```python
from build123d import *

# Parameters (mm, degrees)
SKETCH1_R               = 15.875
SKETCH1_R_2             = 9.5
BOSS_EXTRUDE1_DEPTH     = 6
BOSS_EXTRUDE2_START     = 13.050000011
SKETCH2_R               = 15.875
SKETCH2_R_2             = 9.5
SKETCH2_R_3             = 6.35
BOSS_EXTRUDE2_DEPTH     = 13.050000011
SKETCH3_R               = 1.95
CUT_EXTRUDE1_DEPTH      = 10.16
CUT_EXTRUDE3_REACH      = 39.82
CUT_EXTRUDE3_END_RADIUS = 6.35
BOSS_EXTRUDE3_REACH     = 31.444
SKETCH7_R               = 3.15
CUT_EXTRUDE4_DEPTH      = 31.75
CUT_EXTRUDE5_REACH      = 53.87
CUT_EXTRUDE5_END_RADIUS = 3.15
SKETCH8_R               = 1.95
FILLET1_R               = 9.525


with BuildPart() as part:
    # Sketch1 → Boss-Extrude1 (new body)
    with BuildSketch(Plane(origin=(0, 0, 0), x_dir=(0, 0, -1), z_dir=(1, 0, 0))):
        Circle(SKETCH1_R)
        Circle(SKETCH1_R_2, mode=Mode.SUBTRACT)
    extrude(amount=BOSS_EXTRUDE1_DEPTH)

    # Sketch2 → Boss-Extrude2 (add)
    # profile 1 of 2: a face of its own
    with BuildSketch(Plane.ZY.offset(BOSS_EXTRUDE2_START)):
        Circle(SKETCH2_R)
        with Locations(Location((0, 0, 0), (0, 0, 180))):
            Circle(SKETCH2_R_2, mode=Mode.SUBTRACT)
    # profile 2 of 2: a face of its own
    with BuildSketch(Plane.ZY.offset(BOSS_EXTRUDE2_START)):
        with Locations(Location((0, 0, 0), (0, 0, 180))):
            Circle(SKETCH2_R_2)
        Circle(SKETCH2_R_3, mode=Mode.SUBTRACT)
    extrude(amount=-BOSS_EXTRUDE2_DEPTH)

    # Sketch3 → Cut-Extrude1 (cut)
    with BuildSketch(Plane.ZY.offset(13.050000011)):
        with Locations((0, -12.7)):
            Circle(SKETCH3_R)
        with Locations((0, 12.7)):
            Circle(SKETCH3_R)
    extrude(amount=-CUT_EXTRUDE1_DEPTH, mode=Mode.SUBTRACT)

    # Cut-Extrude3: up to this cylinder (the profile starts outside it)
    cut_extrude3_end = Plane(origin=(-3.525, 0, 0), z_dir=(1, 0, 0)) * Cylinder(CUT_EXTRUDE3_END_RADIUS, 93.34, mode=Mode.PRIVATE)
    # Sketch5 → Cut-Extrude3 (cut, up to the surface)
    with BuildSketch(Plane.XY.offset(-15.875), mode=Mode.PRIVATE) as cut_extrude3_sk1:
        with BuildLine():
            ThreePointArc((-1.575000006, 0), (-3.525000006, 1.95), (-5.475000006, 0))
            Line((-5.475000006, 0), (-1.575000006, 0))
        make_face()
    cut_extrude3_tool1 = extrude(cut_extrude3_sk1.sketch, amount=CUT_EXTRUDE3_REACH, mode=Mode.PRIVATE) - cut_extrude3_end
    add(cut_extrude3_tool1.solids().sort_by_distance((-3.525, 0.827606, -15.875))[0], mode=Mode.SUBTRACT)
    # Sketch5 → Cut-Extrude3 (cut, up to the surface)
    with BuildSketch(Plane.XY.offset(-15.875), mode=Mode.PRIVATE) as cut_extrude3_sk2:
        with BuildLine():
            Line((-1.575000006, 0), (-5.475000006, 0))
            ThreePointArc((-5.475000006, 0), (-3.525000006, -1.95), (-1.575000006, 0))
        make_face()
    cut_extrude3_tool2 = extrude(cut_extrude3_sk2.sketch, amount=CUT_EXTRUDE3_REACH, mode=Mode.PRIVATE) - cut_extrude3_end
    add(cut_extrude3_tool2.solids().sort_by_distance((-3.525, -0.827606, -15.875))[0], mode=Mode.SUBTRACT)
    # Sketch5 → Cut-Extrude3 (cut, up to the surface)
    with BuildSketch(Plane.XY.offset(-15.875), mode=Mode.PRIVATE) as cut_extrude3_sk3:
        with BuildLine():
            ThreePointArc((-1.575000006, 0), (-3.525000006, 1.95), (-5.475000006, 0))
            Line((-5.475000006, 0), (-1.575000006, 0))
        make_face()
    cut_extrude3_tool3 = extrude(cut_extrude3_sk3.sketch, amount=CUT_EXTRUDE3_REACH, mode=Mode.PRIVATE) - cut_extrude3_end
    add(cut_extrude3_tool3.solids().sort_by_distance((-3.525, 0.827606, -15.875))[0], mode=Mode.SUBTRACT)
    # Sketch5 → Cut-Extrude3 (cut, up to the surface)
    with BuildSketch(Plane.XY.offset(-15.875), mode=Mode.PRIVATE) as cut_extrude3_sk4:
        with BuildLine():
            Line((-1.575000006, 0), (-5.475000006, 0))
            ThreePointArc((-5.475000006, 0), (-3.525000006, -1.95), (-1.575000006, 0))
        make_face()
    cut_extrude3_tool4 = extrude(cut_extrude3_sk4.sketch, amount=CUT_EXTRUDE3_REACH, mode=Mode.PRIVATE) - cut_extrude3_end
    add(cut_extrude3_tool4.solids().sort_by_distance((-3.525, -0.827606, -15.875))[0], mode=Mode.SUBTRACT)

    # Boss-Extrude3: up to this face of the body (flat: up to its plane)
    boss_extrude3_end = Plane(part.part.faces().sort_by_distance((6, 0, 15.425987194))[0])
    # Sketch6 → Boss-Extrude3 (add, up to the picked face)
    with BuildSketch(Plane.ZY.offset(13.050000011), mode=Mode.PRIVATE) as boss_extrude3_sk1:
        with BuildLine():
            Line((-15.875, 31.75), (-15.875, 0))
            ThreePointArc((-15.875, 0), (0, 15.875), (15.875, 0))
            Line((15.875, 0), (15.875, 31.75))
            Line((15.875, 31.75), (-15.875, 31.75))
        make_face()
    boss_extrude3_tool1 = split(extrude(boss_extrude3_sk1.sketch, amount=-BOSS_EXTRUDE3_REACH, mode=Mode.PRIVATE), bisect_by=boss_extrude3_end, keep=Keep.BOTH, mode=Mode.PRIVATE)
    add(boss_extrude3_tool1.solids().sort_by(Axis((-13.05, 21.783545, 0), (1, 0, 0)))[0])

    # Sketch7 → Cut-Extrude4 (cut)
    with BuildSketch(Plane.XY.offset(15.875)):
        with Locations((-3.525000006, 21.59)):
            Circle(SKETCH7_R)
    extrude(amount=-CUT_EXTRUDE4_DEPTH, mode=Mode.SUBTRACT)

    # Cut-Extrude5: up to this cylinder (the profile starts outside it)
    cut_extrude5_end = Plane(origin=(-3.525000006, 21.59, 0), z_dir=(0, 0, 1)) * Cylinder(CUT_EXTRUDE5_END_RADIUS, 115.04, mode=Mode.PRIVATE)
    # Sketch8 → Cut-Extrude5 (cut, up to the surface)
    with BuildSketch(Plane(origin=(0, 31.75, 0), x_dir=(1, 0, 0), z_dir=(0, 1, 0)), mode=Mode.PRIVATE) as cut_extrude5_sk1:
        with Locations(Location((-3.525000006, 0, 0), (0, 0, 270))):
            Circle(SKETCH8_R)
    cut_extrude5_tool1 = extrude(cut_extrude5_sk1.sketch, amount=-CUT_EXTRUDE5_REACH, mode=Mode.PRIVATE) - cut_extrude5_end
    add(cut_extrude5_tool1.solids().sort_by_distance((-3.525, 31.75, 0))[0], mode=Mode.SUBTRACT)

    # Fillet1
    # the kernel refuses this fillet: 9.525 mm, written as the material it takes off along each edge
    with BuildSketch(Plane(origin=(6, 31.75, 39.6875), x_dir=(0, -1, 0), z_dir=(0, 0, -1))) as fillet1_piece_1:
        with BuildLine():
            CenterArc((FILLET1_R, FILLET1_R), FILLET1_R, 180, 90)
            Line((0, FILLET1_R), (0, 0))
            Line((0, 0), (FILLET1_R, 0))
        make_face()
    extrude(amount=79.375, mode=Mode.SUBTRACT)
    with BuildSketch(Plane(origin=(-13.050000011, 31.75, 39.6875), x_dir=(0, -1, 0), z_dir=(0, 0, -1))) as fillet1_piece_2:
        with BuildLine():
            CenterArc((FILLET1_R, -FILLET1_R), FILLET1_R, 90, 90)
            Line((0, -FILLET1_R), (0, 0))
            Line((0, 0), (FILLET1_R, 0))
        make_face()
    extrude(amount=79.375, mode=Mode.SUBTRACT)


solid = part.part
```
Model file for the job. Use its own axes, mm. A direction names the side the tool comes from. Coordinates: 2 decimals unless noted, no trailing zeros. Write each loop counter-clockwise with the first axis right and the second up, starting at its lowest first coordinate (ties: lowest second). Pieces come first, ordered by that corner, then holes. Notation, with made-up numbers: (37, -37) - (63, -37) arc R11 ccw to (63, -28) - close; hole circle Ø5 at (-39, 74). An arc over 180 degrees is marked (long way). One line per item, written item: value. Start each with the question number.
1. Flat gauge pins, fed straight in: pin 1 (3 mm diameter, centred on y = 13, z = 0, fed in from -X); pin 2 (11.5 mm diameter, centred on y = 0, z = 0, fed in from +X); pin 3 (7 mm diameter, centred on x = -3.525, y = 21.59, fed in from -Z) (3 decimals); pin 4 (2.5 mm diameter, centred on x = -3.525, z = 0, fed in from +Y). Where does each tip first touch, or does it go through?
2. Slice it at D-D (x = 4.25). Write the cut outline in (y, z) (3 decimals), plus the area to 3 significant figures.
3. Tool access for faces 4 (the flat face through (-2.89, 13, 0)), 5 (the flat face through (0, 2, -6.2)), 6 (the flat face through (-13.05, 8, 0)): list every direction of +Z, -Z, +X, -X, +Y, -Y with a clear straight run to the whole face (end or side of a thin tool).
4. Slice it at A-A (y = 21.59). Write the cut outline in (x, z) (3 decimals), plus the area to 3 significant figures.
5. Probe line 1 (Y direction, x = -2.5, z = -7.5); line 2 (Y direction, x = -2.75, z = -3); line 3 (Y direction, x = 4.5, z = 5). List the from-to ranges inside material, lowest first. Write a range as from..to.
6. Slice it at B-B (z = 0). Write the cut outline in (x, y) (3 decimals).
7. Slice it at C-C (y = 12.7). Write the cut outline in (x, z) (3 decimals).
8. Mould opens along Z. For faces 1 (the flat face through (-4, 16, 15.875)), 2 (the flat face through (-4, 16, -15.875)), 3 (the cylindrical face through (-3.44, 27.96, -1.95)) say: released by +Z, released by -Z, zero draft, split by the parting line, or undercut.
Answers below:
1. pin 1: stops at x = -2.89
1. pin 2: passes through
1. pin 3: stops at z = -15.875
1. pin 4: stops at y = 18.7
2. outline: (0, -15.875) - (27.727, -15.875) - (27.727, 15.875) - (0, 15.875) arc R15.875 ccw to start; hole circle Ø19 at (0, 0)
2. area: 993 mm^2
3. face 4: -X
3. face 5: +X
3. face 6: +Z, -Z, -X, +Y, -Y
4. outline: (-13.05, -15.875) - (-6.675, -15.875) - (-6.675, 15.875) - (-13.05, 15.875) - close; (-0.375, -15.875) - (6, -15.875) - (6, 15.875) - (-0.375, 15.875) - close
4. area: 405 mm^2
5. line 1: y = -13.99..-1.66, 1.66..18.61, 24.57..31.69
5. line 2: y = -15.59..-5.6, 5.6..18.54, 24.64..31.72
5. line 3: y = -15.07..-8.08, 8.08..27.36
6. outline: (-13.05, -15.875) - (6, -15.875) - (6, -9.5) - (0, -9.5) - (0, -6.35) - (-13.05, -6.35) - (-13.05, -10.75) - (-2.89, -10.75) - (-2.89, -14.65) - (-13.05, -14.65) - close; (-13.05, 6.35) - (0, 6.35) - (0, 9.5) - (6, 9.5) - (6, 22.225) arc R9.525 ccw to (-1.575, 31.548) - (-1.575, 24.064) arc R3.15 cw (long way) to (-5.475, 24.064) - (-5.475, 31.548) arc R9.525 ccw to (-13.05, 22.225) - (-13.05, 14.65) - (-2.89, 14.65) - (-2.89, 10.75) - (-13.05, 10.75) - close
7. outline: (-13.05, -15.875) - (6, -15.875) - (6, 15.875) - (-13.05, 15.875) - (-13.05, 1.95) - (-2.89, 1.95) - (-2.89, -1.95) - (-13.05, -1.95) - close
8. face 1: released by +Z
8. face 2: released by -Z
8. face 3: undercut
